```python
from build123d import *

# Parameters (mm, degrees)
SKETCH1_W           = 146.05
SKETCH1_H           = 196.85
BOSS_EXTRUDE1_DEPTH = 76.2
SKETCH2_R           = 3.175
CUT_EXTRUDE1_DEPTH  = 74.5679992
SKETCH3_R           = 3.96875
CUT_EXTRUDE2_DEPTH  = 50.5679964
SKETCH4_R           = 3.175
CUT_EXTRUDE3_DEPTH  = 38.2679956
SKETCH5_R           = 3.96875
CUT_EXTRUDE4_DEPTH  = 6.2680088
SKETCH6_R           = 4
CUT_EXTRUDE5_DEPTH  = 13.0800094


with BuildPart() as part:
    # Sketch1 → Boss-Extrude1 (new body)
    with BuildSketch(Plane(origin=(0, 0, 0), x_dir=(0, 0, -1), z_dir=(1, 0, 0))):
        with Locations((32.001485149, -25.494306931)):
            Rectangle(SKETCH1_W, SKETCH1_H)
    extrude(amount=BOSS_EXTRUDE1_DEPTH)

    # Sketch2 → Cut-Extrude1 (cut)
    with BuildSketch(Plane.XZ.offset(123.919306931)):
        with Locations(Location((15.96, 29.553514851, 0), (0, 0, 270))):
            Circle(SKETCH2_R)
        with Locations(Location((24.84213013, 29.179530425, 0), (0, 0, 270))):
            Circle(SKETCH2_R)
    extrude(amount=-CUT_EXTRUDE1_DEPTH, mode=Mode.SUBTRACT)

    # Sketch3 → Cut-Extrude2 (cut)
    with BuildSketch(Plane.XZ.offset(123.919306931)):
        with Locations(Location((24.840626577, 29.145383002, 0), (0, 0, 270))):
            Circle(SKETCH3_R)
        with Locations(Location((15.96, 29.553514851, 0), (0, 0, 270))):
            Circle(SKETCH3_R)
    extrude(amount=-CUT_EXTRUDE2_DEPTH, mode=Mode.SUBTRACT)

    # Sketch4 → Cut-Extrude3 (cut)
    with BuildSketch(Plane.XZ.offset(123.919306931)):
        with Locations(Location((30.46, -30.446485149, 0), (0, 0, 270))):
            Circle(SKETCH4_R)
    extrude(amount=-CUT_EXTRUDE3_DEPTH, mode=Mode.SUBTRACT)

    # Sketch5 → Cut-Extrude4 (cut)
    with BuildSketch(Plane.XZ.offset(123.919306931)):
        with Locations(Location((30.46, -30.446485149, 0), (0, 0, 270))):
            Circle(SKETCH5_R)
    extrude(amount=-CUT_EXTRUDE4_DEPTH, mode=Mode.SUBTRACT)

    # Sketch6 → Cut-Extrude5 (cut)
    with BuildSketch(Plane(origin=(0, 0, -105.026485149), x_dir=(-1, 0, 0), z_dir=(0, 0, -1))):
        with Locations(Location((-20.96, -56.151306931, 0), (0, 0, 90))):
            Circle(SKETCH6_R)
        with Locations(Location((-20.96, 13.848693069, 0), (0, 0, 90))):
            Circle(SKETCH6_R)
    extrude(amount=-CUT_EXTRUDE5_DEPTH, mode=Mode.SUBTRACT)


solid = part.part
```
Read the model definition and answer for the solid it produces. Units are mm, in the model's axes. A direction names the side the tool comes from. Give positions to 0.01 mm unless a question says otherwise; leave off trailing zeros. Write item = value, one per line. Start each with the question number.
Item 1: Each of these flat-tipped pins is pushed along its axis until it touches: P1, Ø2.5, axis at x = 16, z = 29, coming from the -Y side; P2, Ø6.5, axis at x = 30, z = -30, coming from the -Y side; P3, Ø1.9, axis at x = 29.5, z = -31, coming from the -Y side. Where does it stop, or does it pass through?
Item 2: A tool of negligible diameter and unlimited length cuts with its end or side. For faces 4 (the flat face through (76.2, -24, -31)), 5 (the flat face through (21, -56, -91.946)), 6 (the cylindrical face through (14.028, -61.519, 32.073)), from which of +Z, -Z, +X, -X, +Y, -Y can it reach the whole face along a straight path? Write none if from no direction.
Item 3: The mould has two halves that part along X. Classify faces 1 (the cylindrical face through (22.161, -52.336, -98.578)), 2 (the flat face through (0, -24, -31)), 3 (the flat face through (38, -27, 41.024)): +X half, -X half, draft (parallel to the pull), parting line (faces both ways), or undercut.
Item 4: Find the intervals of material crossed by probe 1 along Z at (x, y) = (25.5, -84), in increasing order. Write a range as [from, to].
Response:
q1.P1 = -49.35
q1.P2 = -117.65
q1.P3 = -85.65
q2.face_4 = +Z, -Z, +X, +Y, -Y
q2.face_5 = -Z
q2.face_6 = -Y
q3.face_1 = undercut
q3.face_2 = -X half
q3.face_3 = draft
q4.probe_1 = [-105.03, 25.23], [33.06, 41.02]
